Study the drawing (mm; zero at the part's minimum x, y, z) and answer. Round coordinates to 2 decimals unless told otherwise and drop trailing zeros. Loops run counter-clockwise (first coordinate to the right, second up) from the corner with the lowest first, then second, coordinate; pieces in that order, holes last. Notation, with made-up numbers: M 65.25,82.25 L 86.25,82.25 A24 ccw 86.25,92.25 Z; hole C 88.25,32.25 d2. An arc over 180 degrees is marked long. Write each question's results on one line, items separated by ' | '.
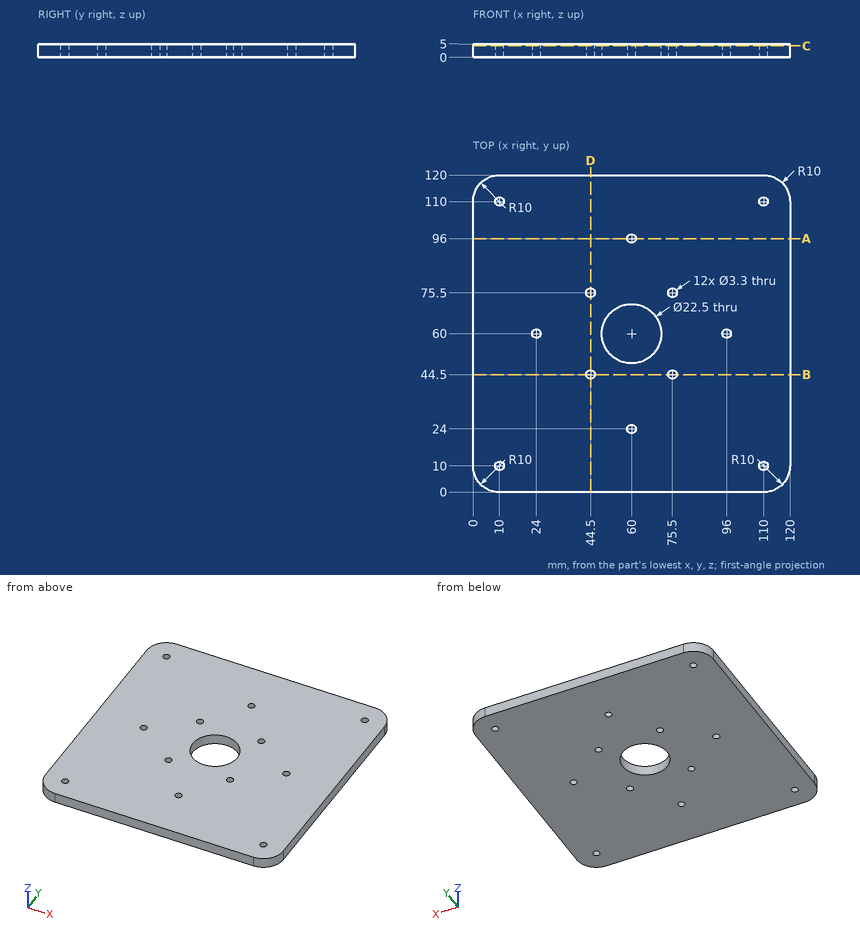
Item 1: The part is cut by section C-C (z = 4.25). State how many separate pieces and enclosed holes the cut face has, plus the area to 3 significant figures.
Outcome:
separate pieces: 1 | enclosed holes: 13 | area: 13,800 mm2
Item 2: Flat-ended cylindrical pins translate along their axes: pin 1 (2 mm diameter, centred on x = 10, y = 10, fed in from +Z); pin 2 (5.5 mm diameter, centred on x = 75.5, y = 75.5, fed in from +Z). Find the tip coordinate at first contact, or state that the pin passes through.
Outcome:
pin 1: passes through | pin 2: stops at z = 5
Item 3: Straight lines are drawn through the part: line 1 (Y direction, x = 10, z = 1.55); line 2 (Y direction, x = 44.5, z = 1.85). For each, find the intervals that lie inside material, in ascending order.
Outcome:
line 1: y = 0 to 8.35, 11.65 to 108.35, 111.65 to 120 | line 2: y = 0 to 42.85, 46.15 to 73.85, 77.15 to 120
Item 4: The part is cut by section A-A (y = 96). Determine the outline of the cut face in (x, z).
Outcome:
outline: M 0,0 L 58.35,0 L 58.35,5 L 0,5 Z; M 61.65,0 L 120,0 L 120,5 L 61.65,5 Z
Item 5: The part is cut by section B-B (y = 44.5). Determine the outline of the cut face in (x, z).
Outcome:
outline: M 0,0 L 42.85,0 L 42.85,5 L 0,5 Z; M 46.15,0 L 73.85,0 L 73.85,5 L 46.15,5 Z; M 77.15,0 L 120,0 L 120,5 L 77.15,5 Z
